Can you work these out from the model? Positions are in its coordinate system, mm. A direction names the side the tool comes from. Round coordinates to 2 decimals unless told otherwise and drop trailing zeros. Order: outer loops, then holes, each group sorted by start corner. A loop starts at its lowest first (then second) coordinate and runs counter-clockwise, first axis right, second up. Notation, with made-up numbers: (75, 49.25) -> (84, 49.25) arc R36 cw to (84, 85.25) -> close; hole circle Ø9 at (49, 57). An arc over 180 degrees is marked (long way). Use a Markdown table: item, result. Add a question column.
Q1. I'm going to push flat-ended pins straight in: pin 1 Ø7.5 at (x, y) = (0, -6) entering from +Z; pin 2 Ø3 at (y, z) = (-6.5, 6) entering from +X; pin 3 Ø1 at (y, z) = (-7, 5) entering from +X. Where does each tip first touch, or does it pass through?
Q2. I need wall thicknesses on line 1 along Y through (x, z) = (0, 5.1); line 2 along Y through (x, z) = (0, 2.8); line 3 along X through (y, z) = (-1.25, 1.5). Which ranges of each line are inside material? Lowest first, please. Write a range as [from, to].
Q3. For faces 4 (the face through (0, 0, 0)), 5 (the face through (9.91, 1.23, 5.77)), which set-ups out of +Z, -Z, +X, -X, +Y, -Y let a thin tool reach every point of the face, with its end or its side?
Q4. If we section it at A-A on x = 0: List the corners of the cut face in (y, z) for me, plus the area to 3 significant figures.
Q5. If we section it at D-D on x = -6: List the corners of the cut face in (y, z) for me.
Q6. If we section it at C-C on z = 1.25: List the corners of the cut face in (x, y) for me.
Q7. We'd pull the mould along X, two halves only. Please class faces 1 (the face through (0, 0, 7)), 2 (the face through (-2.38, -10.74, 3.45)), 3 (the face through (-0.9, 2, 5.8)): +X half, -X half, draft (parallel to the pull), parting line (faces both ways), or undercut.
```python
from build123d import *

# Parameters (mm, degrees)
SKETCH1_R           = 11
BOSS_EXTRUDE1_DEPTH = 7
SKETCH2_R           = 4.1
CUT_EXTRUDE1_DEPTH  = 2.5
SKETCH3_R           = 2.15
CUT_EXTRUDE2_DEPTH  = 10


with BuildPart() as part:
    # Sketch1 → Boss-Extrude1 (new body)
    with BuildSketch(Plane.XY):
        Circle(SKETCH1_R)
    extrude(amount=BOSS_EXTRUDE1_DEPTH)

    # Sketch2 → Cut-Extrude1 (cut)
    with BuildSketch(Plane.XY.offset(7)):
        with Locations((0, 6)):
            Circle(SKETCH2_R)
        with Locations((6, 0)):
            Circle(SKETCH2_R)
        with Locations((0, -6)):
            Circle(SKETCH2_R)
        with Locations((-6, 0)):
            Circle(SKETCH2_R)
    extrude(amount=-CUT_EXTRUDE1_DEPTH, mode=Mode.SUBTRACT)

    # Sketch3 → Cut-Extrude2 (cut)
    with BuildSketch(Plane.XY.offset(4.5)):
        with Locations((0, -6)):
            Circle(SKETCH3_R)
        with Locations((-6, 0)):
            Circle(SKETCH3_R)
        with Locations((0, 6)):
            Circle(SKETCH3_R)
        with Locations((6, 0)):
            Circle(SKETCH3_R)
    extrude(amount=-CUT_EXTRUDE2_DEPTH, mode=Mode.SUBTRACT)


solid = part.part
```
Answer below:
| question | item | result |
|---|---|---|
| 1 | pin 1 | z = 4.5 |
| 1 | pin 2 | x = 9.8 |
| 1 | pin 3 | x = 8.87 |
| 2 | line 1 | [-11, -10.1], [-1.9, 1.9], [10.1, 11] |
| 2 | line 2 | [-11, -8.15], [-3.85, 3.85], [8.15, 11] |
| 2 | line 3 | [-10.93, -7.75], [-4.25, 4.25], [7.75, 10.93] |
| 3 | face 4 | -Z, +X, -X, +Y, -Y |
| 3 | face 5 | +Z |
| 4 | outline | (-11, 0) -> (-8.15, 0) -> (-8.15, 4.5) -> (-10.1, 4.5) -> (-10.1, 7) -> (-11, 7) -> close; (-3.85, 0) -> (3.85, 0) -> (3.85, 4.5) -> (1.9, 4.5) -> (1.9, 7) -> (-1.9, 7) -> (-1.9, 4.5) -> (-3.85, 4.5) -> close; (8.15, 0) -> (11, 0) -> (11, 7) -> (10.1, 7) -> (10.1, 4.5) -> (8.15, 4.5) -> close |
| 4 | area | 74.3 mm² |
| 5 | outline | (-9.22, 0) -> (-2.15, 0) -> (-2.15, 4.5) -> (-4.1, 4.5) -> (-4.1, 7) -> (-9.22, 7) -> close; (2.15, 0) -> (9.22, 0) -> (9.22, 7) -> (4.1, 7) -> (4.1, 4.5) -> (2.15, 4.5) -> close |
| 6 | outline | circle Ø22 at (0, 0); hole circle Ø4.3 at (-6, 0); hole circle Ø4.3 at (0, -6); hole circle Ø4.3 at (0, 6); hole circle Ø4.3 at (6, 0) |
| 7 | face 1 | draft |
| 7 | face 2 | parting line |
| 7 | face 3 | undercut |
